Geometry: final body of the model. Coordinates: model frame, mm. Coordinates: 2 decimals unless noted, no trailing zeros. Order: outer loops, then holes, each group sorted by start corner. A loop starts at its lowest first (then second) coordinate and runs counter-clockwise, first axis right, second up. Notation, with made-up numbers: (-27, -20.75) -> (17, -20.75) arc R22 ccw to (17, -12.75) -> close; hole circle Ø1 at (-27.75, -35.5). An arc over 180 degrees is marked (long way). Use one line per item in the form item = value.
```python
from build123d import *

# Parameters (mm, degrees)
DODANIE_WYCI_GNI_CIE1_DEPTH = 1
SZKIC2_R                    = 1.55
WYTNIJ_WYCI_GNI_CIE1_DEPTH  = 10


with BuildPart() as part:
    # Szkic1 → Dodanie-wyciągnięcie1 (new body)
    with BuildSketch(Plane.XY):
        Polygon((-118.050662271, 36.18823203), (-55.050662271, 36.18823203), (-55.050662271, 43.18823203), (7.949337729, 43.18823203), (7.949337729, 81.18823203), (-118.050662271, 81.18823203), align=None)
    extrude(amount=DODANIE_WYCI_GNI_CIE1_DEPTH)

    # Szkic2 → Wytnij-wyciągnięcie1 (cut)
    with BuildSketch(Plane.XY.offset(1)):
        with Locations((-112.050662271, 77.18823203)):
            Circle(SZKIC2_R)
        with Locations((-112.050662271, 45.18823203)):
            Circle(SZKIC2_R)
        with Locations((-4.050662271, 77.18823203)):
            Circle(SZKIC2_R)
        with Locations((-4.050662271, 45.18823203)):
            Circle(SZKIC2_R)
    extrude(amount=-WYTNIJ_WYCI_GNI_CIE1_DEPTH, mode=Mode.SUBTRACT)


solid = part.part
```
1) Section A-A, the plane z = 0.5. Output: boundary loops of the cut face in (x, y).
Results found:
outline = (-118.05, 36.19) -> (-55.05, 36.19) -> (-55.05, 43.19) -> (7.95, 43.19) -> (7.95, 81.19) -> (-118.05, 81.19) -> close; hole circle Ø3.1 at (-112.05, 45.19); hole circle Ø3.1 at (-112.05, 77.19); hole circle Ø3.1 at (-4.05, 45.19); hole circle Ø3.1 at (-4.05, 77.19)
2) Contact query for flat-ended pins moving along their axis: P1, Ø2.5, axis at x = -112.05, y = 45.19, coming from the +Z side; P2, Ø0.5, axis at y = 41, z = 0.5, coming from the +X side; P3, Ø0.5, axis at x = -37.5, z = 0.5, coming from the -Y side. Output: stop coordinate, or through.
Results found:
P1 = through
P2 = -55.05
P3 = 43.19
3) Section B-B, the plane y = 41.5. Output: boundary loops of the cut face in (x, z).
Results found:
outline = (-118.05, 0) -> (-55.05, 0) -> (-55.05, 1) -> (-118.05, 1) -> close
4) Pull-direction query (Y, two-part tool) for faces 1 (the flat face through (-56, 59, 1)), 2 (the cylindrical face through (-113.6, 45.26, 0.51)); classes: released by +Y, released by -Y, zero draft, split by the parting line, or undercut.
Results found:
face_1 = zero draft
face_2 = undercut
5) Material intervals for probe 1 along X at (y, z) = (78, 0.8); probe 2 along Y at (x, z) = (-7, 0.35); probe 3 along X at (y, z) = (39, 0.8), sorted ascending. Write a range as from..to.
Results found:
probe_1 = -118.05..-113.37, -110.73..-5.37, -2.73..7.95
probe_2 = 43.19..81.19
probe_3 = -118.05..-55.05
6) Section C-C, the plane x = -10.5. Output: boundary loops of the cut face in (y, z), and give its area (3 significant figures).
Results found:
outline = (43.19, 0) -> (81.19, 0) -> (81.19, 1) -> (43.19, 1) -> close
area = 38.0 mm2
